```python
from build123d import *

# Parameters (mm, degrees)
SKETCH1_R           = 40.64
BOSS_EXTRUDE1_DEPTH = 38.100000066
FILLET1_R           = 5
SKETCH2_R           = 3.175
CUT_EXTRUDE1_DEPTH  = 25.4


with BuildPart() as part:
    # Sketch1 → Boss-Extrude1 (new body)
    with BuildSketch(Plane(origin=(0, 0, 0), x_dir=(1, 0, 0), z_dir=(0, 1, 0))):
        with Locations(Location((0, 0, 0), (0, 0, 90))):
            Circle(SKETCH1_R)
    extrude(amount=BOSS_EXTRUDE1_DEPTH)

    # Fillet1
    fillet1_edges = [part.edges().sort_by_distance(p)[0] for p in [
        (0, 0, 40.64),
        (0, 38.100000066, 40.64),
    ]]
    fillet(fillet1_edges, radius=FILLET1_R)

    # Sketch2 → Cut-Extrude1 (cut)
    with BuildSketch(Plane.XZ):
        with Locations(Location((1.587001014, -0.118729115, 0), (0, 0, 270))):
            Circle(SKETCH2_R)
    extrude(amount=-CUT_EXTRUDE1_DEPTH, mode=Mode.SUBTRACT)


solid = part.part
```
Input: part model. Units: mm. Frame: model coordinates. A direction names the side the tool comes from. Coordinates: 2 decimals unless noted, no trailing zeros. Loops run counter-clockwise (first coordinate to the right, second up) from the corner with the lowest first, then second, coordinate; pieces in that order, holes last.
Q1. Contact query for flat-ended pins moving along their axis: pin 1 (10 mm diameter, centred on y = 14, z = -19, fed in from +X); pin 2 (1.5 mm diameter, centred on x = 3.5, y = 28, fed in from +Z); pin 3 (8 mm diameter, centred on y = 29, z = 11.5, fed in from -X). Output: stop coordinate, or through.
Results are:
pin 1: stops at x = 38.15
pin 2: stops at z = 40.55
pin 3: stops at x = -39.94
Q2. Section B-B, the plane x = 0. Return the cut outline in (y, z), and give its area (3 significant figures).
Results are:
outline: (0, -35.64) arc R5 ccw to (5, -40.64) - (33.1, -40.64) arc R5 ccw to (38.1, -35.64) - (38.1, 35.64) arc R5 ccw to (33.1, 40.64) - (5, 40.64) arc R5 ccw to (0, 35.64) - (0, 2.63) - (25.4, 2.63) - (25.4, -2.87) - (0, -2.87) - close
area: 2,940 mm2
Q3. Line query: line 1 along Y through (x, z) = (34, -11); line 2 along X through (y, z) = (24.5, -4.5); line 3 along Z through (x, y) = (37, 27.5). Output: solid intervals per line, ascending.
Results are:
line 1: y = 0 to 38.1
line 2: x = -40.39 to 40.39
line 3: z = -16.81 to 16.81
Q4. Set-up query: faces 1 (the cylindrical face through (4.735, 12.522, 0.295)), 2 (the flat face through (0, 38.1, 0)). Return all of +Z, -Z, +X, -X, +Y, -Y with unobstructed straight access to the full face (end or side cutting, diameter ignored); none if empty.
Results are:
face 1: -Y
face 2: +Z, -Z, +X, -X, +Y
Q5. Section C-C, the plane y = 18.5. Return the cut outline in (x, z) (3 decimals).
Results are:
outline: circle Ø81.28 at (0, 0); hole circle Ø6.35 at (1.587, -0.119)
Q6. Section A-A, the plane z = 0. Return the cut outline in (x, y), and give its area (3 significant figures).
Results are:
outline: (-40.64, 5) arc R5 ccw to (-35.64, 0) - (-1.59, 0) - (-1.59, 25.4) - (4.76, 25.4) - (4.76, 0) - (35.64, 0) arc R5 ccw to (40.64, 5) - (40.64, 33.1) arc R5 ccw to (35.64, 38.1) - (-35.64, 38.1) arc R5 ccw to (-40.64, 33.1) - close
area: 2,910 mm2
Q7. Mould query, pull axis Z, two halves, no side actions, for faces 3 (the flat face through (2, 25.4, 0)), 4 (the flat face through (0, 0, -7)), 5 (the cylindrical face through (-40.294, 18.853, 5.291)). Classes: +Z half, -Z half, draft (parallel to the pull), parting line (faces both ways), or undercut.
Results are:
face 3: undercut
face 4: draft
face 5: parting line
